For this review, take the finished solid that the model builds, in its own axes (mm). Face numbers are marked on the shaded views. Round coordinates to 2 decimals unless told otherwise and drop trailing zeros. Write each loop counter-clockwise with the first axis right and the second up, starting at its lowest first coordinate (ties: lowest second). Pieces come first, ordered by that corner, then holes. Notation, with made-up numbers: M 72,48.25 L 87,48.25 A24 ccw 87,82.25 Z; hole C 35,4.5 d7. An arc over 180 degrees is marked long. Answer in a Markdown table with one row per item.
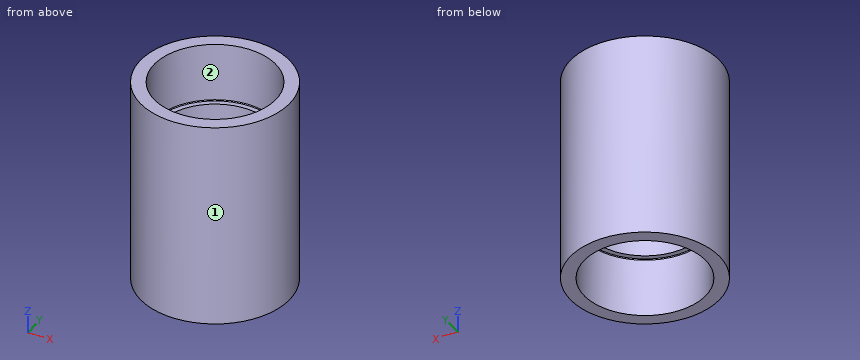
```python
from build123d import *

# Parameters (mm, degrees)
CONG_1_R = 0.4


with BuildPart() as part:
    # Esquisse1 → Révolution1 (revolve)
    with BuildSketch(Plane(origin=(0, 0, 0), x_dir=(0, 0, -1), z_dir=(1, 0, 0)), mode=Mode.PRIVATE) as r_volution1_sk:
        Polygon((-52.5, 38), (52.5, 38), (52.5, 31), (22.5, 31), (22.5, 28), (-22.5, 28), (-22.5, 31), (-52.5, 31), align=None)
    revolve(r_volution1_sk.sketch.rotate(Axis((0, 0, 52.5), (0, 0, -1)), 90), axis=Axis((0, 0, 52.5), (0, 0, -1)))  # turned: the seam where the file's is

    # Congé1
    cong_1_edges = [part.edges().sort_by_distance(p)[0] for p in [
        (-31, 0, 22.5),
        (-31, 0, -22.5),
    ]]
    fillet(cong_1_edges, radius=CONG_1_R)


solid = part.part
```
Q1. Take a section at A-A (y = 0). State the section outline as (x, z) points.
Found:
| item | result |
|---|---|
| outline | M -38,-52.5 L -31,-52.5 L -31,-22.9 A0.4 cw -30.6,-22.5 L -28,-22.5 L -28,22.5 L -30.6,22.5 A0.4 cw -31,22.9 L -31,52.5 L -38,52.5 Z; M 28,-22.5 L 30.6,-22.5 A0.4 cw 31,-22.9 L 31,-52.5 L 38,-52.5 L 38,52.5 L 31,52.5 L 31,22.9 A0.4 cw 30.6,22.5 L 28,22.5 Z |
Q2. Take a section at C-C (z = 33.5). State the section outline as (x, y) points.
Found:
| item | result |
|---|---|
| outline | C 0,0 d76; hole C 0,0 d62 |
Q3. Mouldability with a two-part tool opening along X and no side actions: class the marked faces 1 and 2 as +X half, -X half, draft (parallel to the pull), parting line (faces both ways), or undercut.
Found:
| item | result |
|---|---|
| face 1 | parting line |
| face 2 | undercut |
Q4. For probe 1 along Y at (x, z) = (0, 30.5); probe 2 along Y at (x, z) = (0, -1.5); probe 3 along X at (y, z) = (-13, 6.5), list the stretches that pass through material, from the lowest coordinate up.
Found:
| item | result |
|---|---|
| probe 1 | -38 to -31, 31 to 38 |
| probe 2 | -38 to -28, 28 to 38 |
| probe 3 | -35.71 to -24.8, 24.8 to 35.71 |
Q5. Insertion check: P1, Ø2, axis at y = -9.5, z = 12.5, coming from the -X side; P2, Ø4, axis at x = -7.5, z = -18, coming from the +Y side; P3, Ø12, axis at x = -28, z = -20, coming from the -Y side; P4, Ø10, axis at x = -21.5, y = -1.5, coming from the +Z side. Each pin has a flat end and moves straight along its axis. Give the tip position at first contact, or say it passes through.
Found:
| item | result |
|---|---|
| P1 | x = -37.04 |
| P2 | y = 37.6 |
| P3 | y = -30.98 |
| P4 | through |
Q6. Take a section at D-D (z = 7). State the section outline as (x, y) points.
Found:
| item | result |
|---|---|
| outline | C 0,0 d76; hole C 0,0 d56 |
